from build123d import *

# Parameters (mm, degrees)
BOSS_EXTRUDE1_DEPTH = 2
SKETCH3_R           = 35.55
BOSS_EXTRUDE2_DEPTH = 10
FILLET1_R           = 5
SKETCH4_R           = 1.65
CUT_EXTRUDE1_DEPTH  = 19


with BuildPart() as part:
    # Sketch2 → Boss-Extrude1 (new body)
    with BuildSketch(Plane(origin=(0, 0, 0), x_dir=(1, 0, 0), z_dir=(0, 1, 0))):
        with BuildLine():
            Line((0, 0), (200, 0))
            Line((200, 0), (200, -60))
            Line((200, -60), (0, -60))
            ThreePointArc((0, -60), (-30, -30), (0, 0))
        make_face()
    extrude(amount=BOSS_EXTRUDE1_DEPTH)

    # Sketch3 → Boss-Extrude2 (add)
    with BuildSketch(Plane(origin=(0, 2, 0), x_dir=(1, 0, 0), z_dir=(0, 1, 0))):
        with Locations(Location((0, -30, 0), (0, 0, 57.552333234))):
            Circle(SKETCH3_R)
    extrude(amount=BOSS_EXTRUDE2_DEPTH)

    # Fillet1
    # the kernel refuses this fillet: 5 mm, written as the material it adds along each edge
    with BuildSketch(Plane(origin=(0, 2, 0), x_dir=(0, -1, 0), z_dir=(1, 0, 0))) as fillet1_piece_1_section:
        with BuildLine():
            CenterArc((5, 4), FILLET1_R, 180, 53.130102354)
            Line((0, 4), (0, 0))
            Line((0, 0), (2, 0))
        make_face()
    fillet1_piece_1 = extrude(amount=29.07360742, mode=Mode.PRIVATE)
    fillet1_piece_1 = fillet1_piece_1 & Plane(origin=(0, 2, 30), x_dir=(0.5365290413395907, 0, -0.8438818565410799), z_dir=(0, -1, 0)) * Cylinder(35.55, 75, mode=Mode.PRIVATE)
    add(fillet1_piece_1)
    with BuildSketch(Plane(origin=(29.07360742, 2, 60), x_dir=(0, 0, 1), z_dir=(-1, 0, 0))) as fillet1_piece_2_section:
        with BuildLine():
            CenterArc((4, -5), FILLET1_R, 90, 53.130102354)
            Line((0, -2), (0, 0))
            Line((0, 0), (4, 0))
        make_face()
    fillet1_piece_2 = extrude(amount=29.07360742, mode=Mode.PRIVATE)
    fillet1_piece_2 = fillet1_piece_2 & Plane(origin=(0, 2, 30), x_dir=(0.5365290413395907, 0, -0.8438818565410799), z_dir=(0, -1, 0)) * Cylinder(35.55, 75, mode=Mode.PRIVATE)
    add(fillet1_piece_2)
    with BuildSketch(Plane(origin=(0, 2, 30), x_dir=(0, 0, 1), z_dir=(1, 0, 0))) as fillet1_piece_3:
        with BuildLine():
            CenterArc((34, 5), FILLET1_R, 216.869897646, 53.130102354)
            Line((34, 0), (30, 0))
            Line((30, 0), (30, 2))
        make_face()
    revolve(axis=Axis((0, 2, 30), (0, -1, 0)), revolution_arc=180)

    # Sketch4 → Cut-Extrude1 (cut)
    with BuildSketch(Plane(origin=(0, 12, 0), x_dir=(1, 0, 0), z_dir=(0, 1, 0))):
        with Locations(Location((0, -5, 0), (0, 0, 270))):
            Circle(SKETCH4_R)
        with Locations(Location((0, -55, 0), (0, 0, 270))):
            Circle(SKETCH4_R)
        with Locations(Location((-20.478801107, -15.660589091, 0), (0, 0, 270))):
            Circle(SKETCH4_R)
        with Locations(Location((-20.478801107, -44.339410909, 0), (0, 0, 270))):
            Circle(SKETCH4_R)
        with Locations(Location((20.478801107, -15.660589091, 0), (0, 0, 270))):
            Circle(SKETCH4_R)
        with Locations(Location((20.478801107, -44.339410909, 0), (0, 0, 270))):
            Circle(SKETCH4_R)
    extrude(amount=-CUT_EXTRUDE1_DEPTH, mode=Mode.SUBTRACT)


solid = part.part
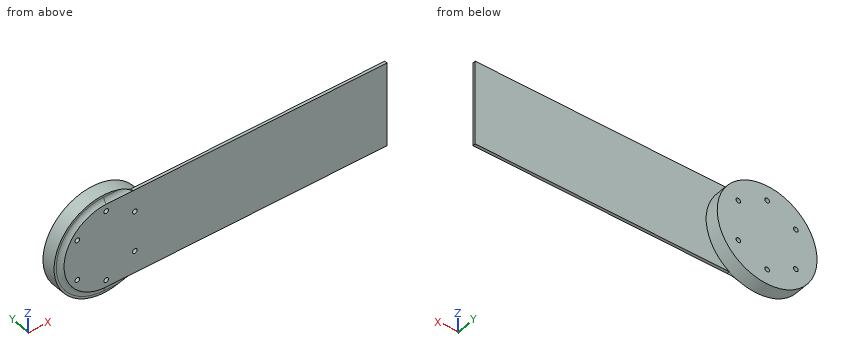
Can you work these out from the model? Positions are in its coordinate system, mm. Give positions to 0.01 mm unless a question says otherwise; leave off trailing zeros. Loops run counter-clockwise (first coordinate to the right, second up) from the corner with the lowest first, then second, coordinate; pieces in that order, holes last. Notation, with made-up numbers: M -16,-23.75 L 22,-23.75 A20 cw 22,-15.75 Z; hole C 78,67.25 d3. An arc over 180 degrees is marked long. One line per item, written item: value. Start each with the question number.
1) If we section it at A-A, the plane z = 30: Write out the boundary of the cut face in (x, y), and give its area (3 significant figures).
2) If we section it at B-B, the plane y = 4: Write out the boundary of the cut face in (x, z).
3) If I drill on line 1 (Z direction, x = -21.5, y = 7.5); line 2 (X direction, y = 3.75, z = 30.5); line 3 (Y direction, x = 173, z = 40), over which ranges is the centre line in solid material (lowest first)? Write a range as [from, to].
4) I'm going to push flat-ended pins straight in: pin 1 (0.6 mm diameter, centred on x = 134, y = 1.5, fed in from -Z); pin 2 (4.5 mm diameter, centred on x = 20.48, z = 44.34, fed in from -Y); pin 3 (2 mm diameter, centred on y = 8.5, z = 33.5, fed in from -X); pin 4 (4 mm diameter, centred on y = 9, z = 57, fed in from -X). Where does each tip first touch, or does it pass through?
5) If we section it at C-C, the plane x = 112: Write out the boundary of the cut face in (y, z).
Completed:
1. outline: M -35.55,2 L -34,2 A5 cw -30,0 L 200,0 L 200,2 L 35.55,2 L 35.55,12 L -35.55,12 Z
1. area: 1,170 mm^2
2. outline: C 0,30 d71.1; hole C -20.48,15.66 d3.3; hole C -20.48,44.34 d3.3; hole C 0,5 d3.3; hole C 0,55 d3.3; hole C 20.48,15.66 d3.3; hole C 20.48,44.34 d3.3
3. line 1: z = [1.69, 14.36], [16.96, 43.04], [45.64, 58.31]
3. line 2: x = [-35.55, 35.55]
3. line 3: y = [0, 2]
4. pin 1: stops at z = 0
4. pin 2: stops at y = 0
4. pin 3: stops at x = -35.46
4. pin 4: stops at x = -25.27
5. outline: M 0,0 L 2,0 L 2,60 L 0,60 Z
